Could you check a few things on this drawing? It's one solid part, dimensions in mm from its lowest x, y, z. A direction names the side the tool comes from. Give positions to 0.01 mm unless a question says otherwise; leave off trailing zeros. Write each loop counter-clockwise with the first axis right and the second up, starting at its lowest first coordinate (ties: lowest second). Pieces come first, ordered by that corner, then holes. Notation, with made-up numbers: M -40,37.5 L 18,37.5 A34 cw 18,71.5 Z; hole C 77,87.25 d2. An arc over 180 degrees is marked long. Write each question's results on one line, items separated by ' | '.
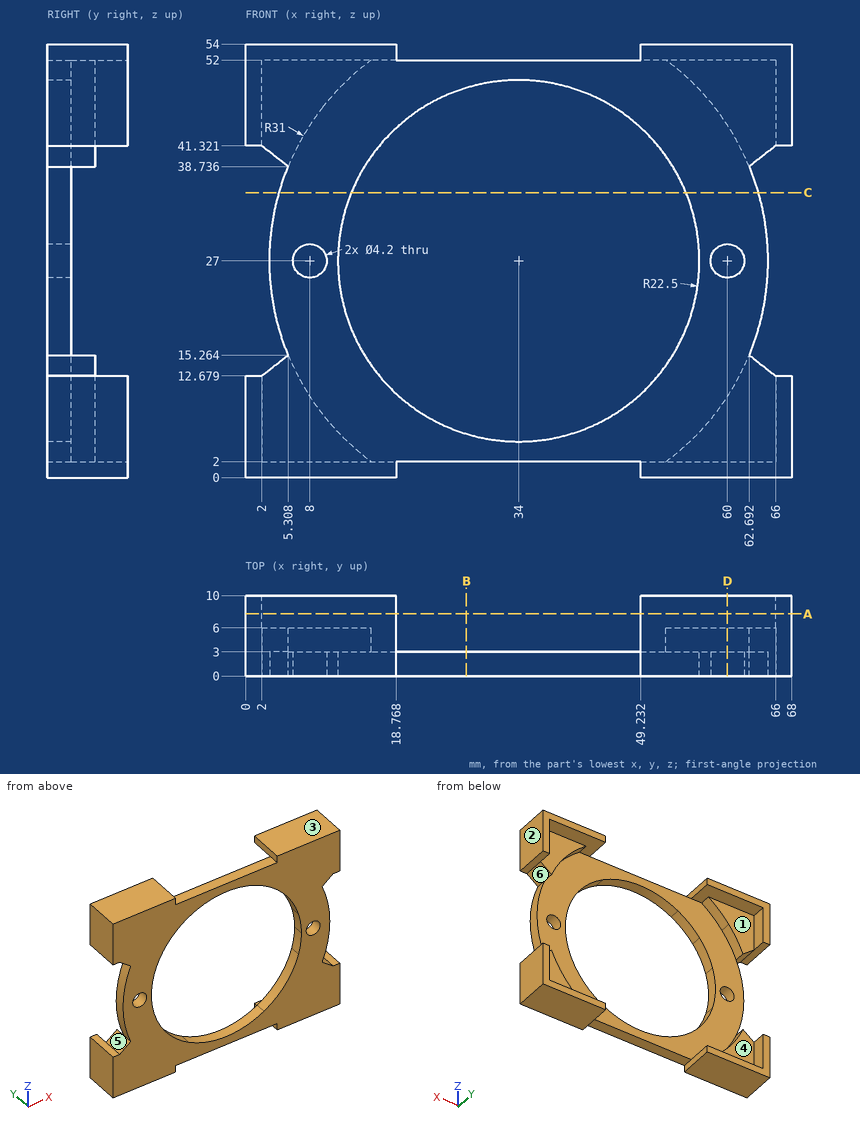
Item 1: I want a section at D-D, the plane x = 60. Please give me the cut outline in (y, z).
Geometry says:
outline: M 0,0 L 10,0 L 10,2 L 6,2 L 6,10.12 L 3,10.12 L 3,24.9 L 0,24.9 Z; M 0,29.1 L 3,29.1 L 3,43.88 L 6,43.88 L 6,52 L 10,52 L 10,54 L 0,54 Z
Item 2: If I drill on line 1 (X direction, y = 0.9, z = 27); line 2 (X direction, y = 6.5, z = 45); line 3 (Y direction, x = 8, z = 44), over which ranges is the centre line in solid material (lowest first)? Write a range as from..to.
Geometry says:
line 1: x = 3..5.9, 10.1..11.5, 56.5..57.9, 62.1..65 | line 2: x = 0..2, 66..68 | line 3: y = 0..6
Item 3: For the marked faces 4, 5 and 6, which set-ups out of +Z, -Z, +X, -X, +Y, -Y let a thin tool reach every point of the face, with its end or its side?
Geometry says:
face 4: +Y | face 5: -X, +Y, -Y | face 6: +X, +Y, -Y
Item 4: I want a section at C-C, the plane z = 35.5. Please give me the cut outline in (x, y).
Geometry says:
outline: M 4.19,0 L 13.17,0 L 13.17,3 L 4.19,3 Z; M 54.83,0 L 63.81,0 L 63.81,3 L 54.83,3 Z
Item 5: I want a section at B-B, the plane x = 27.5. Please give me the cut outline in (y, z).
Geometry says:
outline: M 0,2 L 3,2 L 3,5.46 L 0,5.46 Z; M 0,48.54 L 3,48.54 L 3,52 L 0,52 Z
Item 6: I'm going to push flat-ended pins straight in: pin 1 (5.5 mm diameter, centred on x = 8, z = 27, fed in from +Y); pin 2 (0.9 mm diameter, centred on x = 41, y = 2, fed in from +Z); pin 3 (6.5 mm diameter, centred on x = 58.5, z = 46, fed in from +Y); pin 4 (1.5 mm diameter, centred on y = 4.5, z = 30.5, fed in from +X). Where does each tip first touch, or does it pass through?
Geometry says:
pin 1: stops at y = 3 | pin 2: stops at z = 52 | pin 3: stops at y = 6 | pin 4: passes through
Item 7: Thinking about a two-plate mould opening in X: for the marked faces 1, 2 and 3, which applies, +X half, -X half, draft (parallel to the pull), parting line (faces both ways), or undercut?
Geometry says:
face 1: undercut | face 2: +X half | face 3: draft
Item 8: I want a section at A-A, the plane y = 7.75. Please give me the cut outline in (x, z).
Geometry says:
outline: M 0,0 L 18.77,0 L 18.77,2 L 2,2 L 2,12.68 L 0,12.68 Z; M 0,41.32 L 2,41.32 L 2,52 L 18.77,52 L 18.77,54 L 0,54 Z; M 49.23,0 L 68,0 L 68,12.68 L 66,12.68 L 66,2 L 49.23,2 Z; M 49.23,52 L 66,52 L 66,41.32 L 68,41.32 L 68,54 L 49.23,54 Z
